Autodesk Inventor part; units mm, degrees
ref_plane "YZ Plane" through (0, 0, 0) normal (1, 0, 0) x (0, 1, 0)
ref_plane "XZ Plane" through (0, 0, 0) normal (0, 1, 0) x (-1, 0, 0)
ref_plane "XY Plane" through (0, 0, 0) normal (0, 0, 1) x (1, 0, 0)
sketch "スケッチ1" plane through (0, 0, 0) normal (0, 1, 0) x (-1, 0, 0)
  line L0 (-3, 0.3) -> (-3, 3.7)
  line L1 (-3.3, 4) -> (-3.7, 4)
  line L2 (-4, 3) -> (-4, 1)
  line L3 (-4, 1) -> (-6, 1)
  line L4 (-6, 1) -> (-6, 0)
  line L5 (-6, 0) -> (-3.3, 0)
  line L6 (-3, 3.7) -> (-3.3, 4)
  line L7 (-3, 0.3) -> (-3.3, 0)
  line L8 (-3.7, 4) -> (-4, 3)
  line L9 (0, -0.8) -> (0, 4.8)
  point P0 (0, 0)
  point P1 (-3, 0)
  point P2 (-3, 4)
  point P3 (-4, 4)
  dimension "d2" = 1
  dimension "d9" = 1
  dimension "d11" = 6
  dimension "d12" = 8
  dimension "d13" = 12
  dimension "d14" = 0.3
  dimension "d15" = 0.3
  dimension "d16" = 0.3
  dimension "d17" = 0.3
  dimension "d18" = 0.3
  dimension "d19" = 4
revolve "回転1" add sketch "スケッチ1" angle 360 about axis through (0, 0, -10) along (0, 0, 1)
equation "\"d15\" = d14"
equation "\"d16\" = d14"
equation "\"d17\" = d16"
equation "\"d18\" = d14"
properties part number "80F-0603"
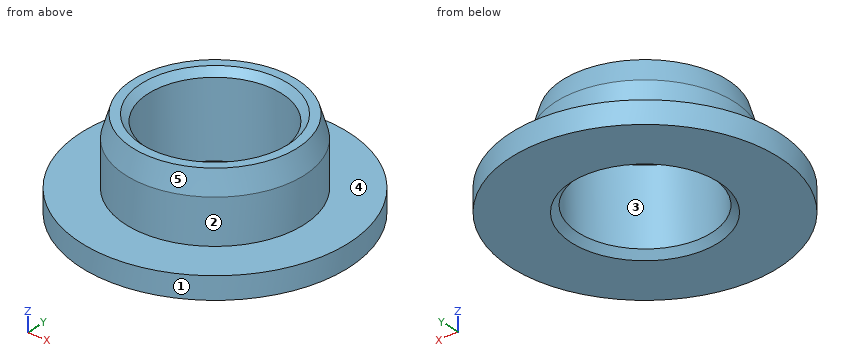
Work out the finished part from the listing and answer in its coordinate system (mm). Face numbers are marked on the shaded views. A direction names the side the tool comes from. Give positions to 0.01 mm unless a question says otherwise; leave off trailing zeros. Order: outer loops, then holes, each group sorted by start corner. A loop starts at its lowest first (then second) coordinate and runs counter-clockwise, first axis right, second up.
1. Each of these flat-tipped pins is pushed along its axis until it touches: P1, Ø3.5, axis at x = 1, y = 0, coming from the +Z side; P2, Ø1.5, axis at y = 4, z = 2, coming from the -X side; P3, Ø4, axis at x = 0.5, y = -1, coming from the +Z side. Where does it stop, or does it pass through?
Result sheet:
P1: passes through
P2: stops at x = -2.33
P3: stops at z = 3.82
2. Straight lines are drawn through the part: L1, parallel to Y at x = 0, z = 1.7; L2, parallel to Z at x = 2, y = -5.5; L3, parallel to Y at x = -0.75, z = 1.2. For each, find the intervals that lie inside material, in ascending order.
Result sheet:
L1: y = -4 to -3, 3 to 4
L2: z = 0 to 1
L3: y = -3.93 to -2.9, 2.9 to 3.93
3. Section C-C, the plane z = 0.55 is taken. Determine the outline of the cut face in (x, y).
Result sheet:
outline: circle Ø12 at (0, 0); hole circle Ø6 at (0, 0)
4. Section D-D, the plane y = -4.5 is taken. Determine the outline of the cut face in (x, z), and give its area (3 significant figures).
Result sheet:
outline: (-3.97, 0) - (3.97, 0) - (3.97, 1) - (-3.97, 1) - close
area: 7.94 mm2
5. The mould has two halves that part along Y. Classify the marked faces 3, 4 and 5: released by +Y, released by -Y, zero draft, split by the parting line, or undercut.
Result sheet:
face 3: undercut
face 4: zero draft
face 5: split by the parting line
6. For the marked faces 1 and 2, determine the directions among +Z, -Z, +X, -X, +Y, -Y from which every point of the face is accessible in a straight line to the end or side of a thin tool.
Result sheet:
face 1: +Z, -Z
face 2: +Z
7. Section A-A, the plane y = 0 is taken. Determine the outline of the cut face in (x, z).
Result sheet:
outline: (-6, 0) - (-3.3, 0) - (-3, 0.3) - (-3, 3.7) - (-3.3, 4) - (-3.7, 4) - (-4, 3) - (-4, 1) - (-6, 1) - close; (3, 0.3) - (3.3, 0) - (6, 0) - (6, 1) - (4, 1) - (4, 3) - (3.7, 4) - (3.3, 4) - (3, 3.7) - close
